Autodesk Inventor part; units mm, degrees
ref_plane "YZ Plane" through (0, 0, 0) normal (1, 0, 0) x (0, 1, 0)
ref_plane "XZ Plane" through (0, 0, 0) normal (0, 1, 0) x (-1, 0, 0)
ref_plane "XY Plane" through (0, 0, 0) normal (0, 0, 1) x (1, 0, 0)
sketch "스케치1" plane through (0, 0, 0) normal (0, 0, 1) x (1, 0, 0)
  line L0 (-48, 7) -> (48, 7)
  line L1 (48, 7) -> (48, -7)
  line L2 (48, -7) -> (-48, -7)
  line L3 (-48, -7) -> (-48, 7)
  line L4 (-48, 7) -> (48, -7) construction
  line L5 (48, 7) -> (-48, -7) construction
  point P0 (0, 0)
  dimension "d0" = 96
  dimension "d1" = 14
extrude "돌출1" add sketch "스케치1" along normal blind 4
sketch "스케치2" plane through (0, 0, 4) normal (0, 0, 1) x (1, 0, 0)
  line L0 (-48, -7) -> (48, -7)
  line L1 (48, -7) -> (48, 7)
  line L2 (48, 7) -> (-48, 7)
  line L3 (-48, 7) -> (-48, -7)
  circle A0 centre (-42.1, 0) radius 2.1
  circle A1 centre (42.1, 0) radius 2.1
  point P0 (0, 0)
  dimension "d4" = 4.2
  dimension "d5" = 4.2
  dimension "d6" = 84.2
  dimension "d7" = 5.9
  dimension "d10" = 7
extrude "돌출2" cut sketch "스케치2" against normal blind 4 contours A0 | A1
fillet "모깎기1" radius 2 4 edges at (48, 7, 2) (48, -7, 2) (-48, 7, 2) (-48, -7, 2)
sketch "스케치3" plane through (0, 0, 4) normal (0, 0, 1) x (1, 0, 0)
  circle A0 centre (0, 0) radius 1.6
  dimension "d12" = 3.2
extrude "돌출3" cut sketch "스케치3" against normal blind 4
sketch "스케치5" plane through (0, 0, 4) normal (0, 0, 1) x (1, 0, 0)
  circle A0 centre (0, 0) radius 1.6
  arc A1 (-48, -5) -> (-46, -7) centre (-46, -5) ccw
  line L0 (-46, -7) -> (46, -7)
  arc A2 (46, -7) -> (48, -5) centre (46, -5) ccw
  line L1 (48, -5) -> (48, 5)
  arc A3 (48, 5) -> (46, 7) centre (46, 5) ccw
  line L2 (46, 7) -> (-46, 7)
  arc A4 (-46, 7) -> (-48, 5) centre (-46, 5) ccw
  line L3 (-48, 5) -> (-48, -5)
  circle A5 centre (42.1, 0) radius 2.1
  circle A6 centre (-42.1, 0) radius 2.1
  arc A7 (-46, 7) -> (-48, 5) centre (-46, 5) ccw
  line L4 (-48, 5) -> (-48, 20)
  line L5 (-44, 24) -> (44, 24)
  arc A8 (48, 5) -> (46, 7) centre (46, 5) ccw
  line L6 (48, 20) -> (48, 5)
  arc A9 (-44, 24) -> (-48, 20) centre (-44, 20) ccw
  arc A10 (48, 20) -> (44, 24) centre (44, 20) ccw
  point P0 (-48, 24)
  point P1 (48, 24)
  dimension "d18" = 19
  dimension "d21" = 4
sketch "스케치6" plane through (0, 0, 4) normal (0, 0, 1) x (1, 0, 0)
  circle A0 centre (0, 0) radius 1.6
  arc A1 (-48, -5) -> (-46, -7) centre (-46, -5) ccw
  line L0 (-46, -7) -> (46, -7)
  arc A2 (46, -7) -> (48, -5) centre (46, -5) ccw
  line L1 (48, -5) -> (48, 20)
  arc A3 (48, 20) -> (44, 24) centre (44, 20) ccw
  line L2 (44, 24) -> (-44, 24)
  arc A4 (-44, 24) -> (-48, 20) centre (-44, 20) ccw
  line L3 (-48, 20) -> (-48, -5)
  circle A5 centre (42.1, 0) radius 2.1
  circle A6 centre (-42.1, 0) radius 2.1
  line L4 (48, -5) -> (48, 20)
  line L5 (-48, 23.602) -> (48, 23.602)
  line L6 (48, 23.602) -> (48, 18)
  line L7 (48, 18) -> (-48, 18)
  line L8 (-48, 18) -> (-48, 23.602)
  circle A7 centre (0, 20.4) radius 1.6
  circle A8 centre (-42.1, 20.4) radius 1.6
  circle A9 centre (42.1, 20.4) radius 1.6
  dimension "d23" = 3.2
  dimension "d24" = 3.2
  dimension "d35" = 3.6
sketch "스케치8" plane through (0, 0, 0) normal (0, 0, -1) x (-1, 0, 0)
  circle A0 centre (-42.1, 20.4) radius 1.6
  circle A1 centre (0, 20.4) radius 1.6
  circle A2 centre (42.1, 20.4) radius 1.6
  circle A3 centre (0, 0) radius 1.6
  circle A4 centre (-42.1, 0) radius 2.1
  circle A5 centre (42.1, 0) radius 2.1
  arc A6 (46, -7) -> (48, -5) centre (46, -5) ccw
  line L0 (48, 20) -> (48, -5)
  arc A7 (48, 20) -> (44, 24) centre (44, 20) ccw
  line L1 (44, 24) -> (-44, 24)
  arc A8 (-44, 24) -> (-48, 20) centre (-44, 20) ccw
  line L2 (-48, 20) -> (-48, -5)
  arc A9 (-48, -5) -> (-46, -7) centre (-46, -5) ccw
  line L3 (46, -7) -> (-46, -7)
  line L4 (-48, 24) -> (-18, 24)
  line L5 (-18, 24) -> (-18, 9)
  line L6 (-18, 9) -> (-48, 9)
  line L7 (-48, 9) -> (-48, 24)
  point P0 (-44, 24)
  dimension "d27" = 30
  dimension "d28" = 15
sketch "스케치10" plane through (0, 0, 0) normal (0, 0, -1) x (-1, 0, 0)
  arc A0 (-45, 9) -> (-48, 6) centre (-45, 6) ccw
  line L0 (-48, 6) -> (-48, -5)
  arc A1 (-48, -5) -> (-46, -7) centre (-46, -5) ccw
  line L1 (46, -7) -> (-46, -7)
  arc A2 (46, -7) -> (48, -5) centre (46, -5) ccw
  line L2 (48, 20) -> (48, -5)
  arc A3 (48, 20) -> (44, 24) centre (44, 20) ccw
  line L3 (44, 24) -> (-15, 24)
  arc A4 (-15, 24) -> (-18, 21) centre (-15, 21) ccw
  line L4 (-18, 21) -> (-18, 12)
  arc A5 (-21, 9) -> (-18, 12) centre (-21, 12) ccw
  line L5 (-21, 9) -> (-45, 9)
  circle A6 centre (42.1, 0) radius 2.1
  circle A7 centre (-42.1, 0) radius 2.1
  circle A8 centre (0, 0) radius 1.6
  circle A9 centre (42.1, 20.4) radius 1.6
  circle A10 centre (0, 20.4) radius 1.6
  circle A11 centre (21.05, 20.4) radius 1.6
  dimension "d32" = 21.05
properties part number "축지지프레임" material "알루미늄 6061"
Geometry: final body of the model. Coordinates: model frame, mm. Round coordinates to 2 decimals unless told otherwise and drop trailing zeros. Order: outer loops, then holes, each group sorted by start corner. A loop starts at its lowest first (then second) coordinate and runs counter-clockwise, first axis right, second up. Notation, with made-up numbers: (41, 78.25) -> (53, 78.25) arc R34 ccw to (53, 114.25) -> close; hole circle Ø2 at (89.5, -6). An arc over 180 degrees is marked (long way). Put each result on its own line as item: value. Start each with the question number.
Q1. Section A-A on x = 42.1. Return the cut outline in (y, z).
Q2. Section D-D on x = 0. Return the cut outline in (y, z).
Q3. Section C-C on z = 2.05. Return the cut outline in (x, y).
Q4. Section B-B on y = 0. Return the cut outline in (x, z), and give its area (3 significant figures).
Q5. Line query: probe 1 along Y at (x, z) = (42.1, 1.5); probe 2 along X at (y, z) = (0.5, 3.1); probe 3 along Y at (x, z) = (0, 1). Output: solid intervals per line, ascending.
Q6. Pull-direction query (X, two-part tool) for faces 1 (the cylindrical face through (-1.27, -0.97, 2.03)), 2 (the flat face through (-1, 7, 2)), 3 (the flat face through (48, 0, 2)), 4 (the cylindrical face through (40, 0, 2)); classes: +X half, -X half, draft (parallel to the pull), parting line (faces both ways), or undercut.
Ans:
1. outline: (-7, 0) -> (-2.1, 0) -> (-2.1, 4) -> (-7, 4) -> close; (2.1, 0) -> (7, 0) -> (7, 4) -> (2.1, 4) -> close
2. outline: (-7, 0) -> (-1.6, 0) -> (-1.6, 4) -> (-7, 4) -> close; (1.6, 0) -> (7, 0) -> (7, 4) -> (1.6, 4) -> close
3. outline: (-48, -5) arc R2 ccw to (-46, -7) -> (46, -7) arc R2 ccw to (48, -5) -> (48, 5) arc R2 ccw to (46, 7) -> (-46, 7) arc R2 ccw to (-48, 5) -> close; hole circle Ø4.2 at (-42.1, 0); hole circle Ø3.2 at (0, 0); hole circle Ø4.2 at (42.1, 0)
4. outline: (-48, 0) -> (-44.2, 0) -> (-44.2, 4) -> (-48, 4) -> close; (-40, 0) -> (-1.6, 0) -> (-1.6, 4) -> (-40, 4) -> close; (1.6, 0) -> (40, 0) -> (40, 4) -> (1.6, 4) -> close; (44.2, 0) -> (48, 0) -> (48, 4) -> (44.2, 4) -> close
4. area: 338 mm2
5. probe 1: y = -7 to -2.1, 2.1 to 7
5. probe 2: x = -48 to -44.14, -40.06 to -1.52, 1.52 to 40.06, 44.14 to 48
5. probe 3: y = -7 to -1.6, 1.6 to 7
6. face 1: undercut
6. face 2: draft
6. face 3: +X half
6. face 4: undercut
